from build123d import *

# Parameters (mm, degrees)
SKETCH_5_W           = 60
SKETCH_5_H           = 115
EXTRUDE_2_DEPTH      = 20
SKETCH_1_R           = 1.05
CUT_EXTRUDE_4_DEPTH  = 20
SKETCH_6_R           = 5
EXTRUDE_3_DEPTH      = 13
SKETCH_22_W          = 21
SKETCH_22_H          = 21
CUT_EXTRUDE_9_DEPTH  = 17
SKETCH_22_6_W        = 21
SKETCH_22_6_H        = 21
CUT_EXTRUDE_10_DEPTH = 17


with BuildPart() as part:
    # Sketch 5 → Extrude 2 (new body)
    with BuildSketch(Plane.XY):
        with Locations((85.095319229, -3)):
            Rectangle(SKETCH_5_W, SKETCH_5_H)
    extrude(amount=EXTRUDE_2_DEPTH)

    # Sketch 1 → Cut-Extrude 4 (cut)
    with BuildSketch(Plane.XY):
        with Locations((59.19, 1.7)):
            Circle(SKETCH_1_R)
        with Locations((106.81, 1.7)):
            Circle(SKETCH_1_R)
        with Locations((106.81, -7.7)):
            Circle(SKETCH_1_R)
        with Locations((59.19, -7.7)):
            Circle(SKETCH_1_R)
        Polygon((55, -3), (55, 0), (62, 0), (62, 7.5), (104, 7.5), (104, -13.5), (62, -13.5), (62, -6), (55, -6), align=None)
    extrude(amount=CUT_EXTRUDE_4_DEPTH, mode=Mode.SUBTRACT)

    # Sketch 6 → Extrude 3 (add)
    with BuildSketch(Plane(origin=(115, 0, 0), x_dir=(0, 0, -1), z_dir=(1, 0, 0))):
        with Locations((-10, 44.5)):
            Circle(SKETCH_6_R)
        with Locations((-10, 29.5)):
            Circle(SKETCH_6_R)
        with Locations((-10, -35.5)):
            Circle(SKETCH_6_R)
        with Locations((-10, -50.5)):
            Circle(SKETCH_6_R)
    extrude(amount=EXTRUDE_3_DEPTH)

    # Sketch 22 → Cut-Extrude 9 (cut)
    with BuildSketch(Plane.XY):
        with Locations((85, 37.5)):
            Rectangle(SKETCH_22_W, SKETCH_22_H)
    extrude(amount=CUT_EXTRUDE_9_DEPTH, mode=Mode.SUBTRACT)

    # Sketch 22_6 → Cut-Extrude 10 (cut)
    with BuildSketch(Plane.XY):
        with Locations((85, -43.5)):
            Rectangle(SKETCH_22_6_W, SKETCH_22_6_H)
    extrude(amount=CUT_EXTRUDE_10_DEPTH, mode=Mode.SUBTRACT)


solid = part.part
Verification items for the finished model (mm, model axes). A direction names the side the tool comes from. Coordinates: 2 decimals unless noted, no trailing zeros. Order: outer loops, then holes, each group sorted by start corner. A loop starts at its lowest first (then second) coordinate and runs counter-clockwise, first axis right, second up. Notation, with made-up numbers: M -24,2 L -4,2 A22 cw -4,24 Z; hole C 11.25,54 d7. An arc over 180 degrees is marked long. Write each question's results on one line, items separated by ' | '.
1) Section check B-B on z = 3.75. Record the cut outline in (x, y), plus the area to 3 significant figures.
Solved:
outline: M 55.1,-60.5 L 115.1,-60.5 L 115.1,54.5 L 55.1,54.5 L 55.1,0 L 62,0 L 62,7.5 L 104,7.5 L 104,-13.5 L 62,-13.5 L 62,-6 L 55.1,-6 Z; hole C 59.19,-7.7 d2.1; hole C 59.19,1.7 d2.1; hole M 74.5,-54 L 95.5,-54 L 95.5,-33 L 74.5,-33 Z; hole M 74.5,27 L 95.5,27 L 95.5,48 L 74.5,48 Z; hole C 106.81,-7.7 d2.1; hole C 106.81,1.7 d2.1 | area: 5,080 mm²
2) Gauge pin test, flat ends, axial feed: pin 1 Ø2 at (y, z) = (-9, 12) entering from +X; pin 2 Ø5 at (x, y) = (93.5, -45) entering from -Z; pin 3 Ø10 at (x, y) = (74.5, -4.5) entering from -Z. Record the tip position at first contact, or that the pin passes through.
Solved:
pin 1: stops at x = 115.1 | pin 2: stops at z = 0 | pin 3: passes through
3) Release check for a two-part mould opening along Y. For faces 1 (the face through (58.14, -7.65, 9.86)), 2 (the face through (74.5, 37, 8)), 3 (the face through (85, 54.5, 10)), 4 (the face through (128, -50, 10)) record: pulls with the +Y half, pulls with the -Y half, needs draft (parallel to the pull), parting line crosses it, or undercut.
Solved:
face 1: undercut | face 2: undercut | face 3: pulls with the +Y half | face 4: needs draft
4) Section check D-D on z = 13. Give the number of separate pieces and of enclosed holes in the cut face, plus the area to 3 significant figures.
Solved:
separate pieces: 1 | enclosed holes: 6 | area: 5,490 mm²
5) Access from +Z, -Z, +X, -X, +Y, -Y to the whole of each face (thin tool, end or side, straight path). Record for faces 5 (the face through (83, -13.5, 10)), 6 (the face through (58, 0, 10)), 7 (the face through (95.5, -44, 8)), 8 (the face through (121.457, 48.716, 7.312)).
Solved:
face 5: +Z, -Z | face 6: +Z, -Z, -X | face 7: -Z | face 8: +X
6) Section check A-A on x = 90.5. Record the cut outline in (y, z), plus the area to 3 significant figures.
Solved:
outline: M -60.5,0 L -54,0 L -54,17 L -33,17 L -33,0 L -13.5,0 L -13.5,20 L -60.5,20 Z; M 7.5,0 L 27,0 L 27,17 L 48,17 L 48,0 L 54.5,0 L 54.5,20 L 7.5,20 Z | area: 1,170 mm²
7) Scan lines: line 1 along Y through (x, z) = (59.19, 15.75); line 2 along Y through (x, z) = (84.5, 11.5); line 3 along Y through (x, z) = (106.81, 4.25). Record each from-to range of solid material in increasing order. Write a range as [from, to].
Solved:
line 1: y = [-60.5, -8.75], [-6.65, -6], [0, 0.65], [2.75, 54.5] | line 2: y = [-60.5, -54], [-33, -13.5], [7.5, 27], [48, 54.5] | line 3: y = [-60.5, -8.75], [-6.65, 0.65], [2.75, 54.5]
8) Section check C-C on y = 29.5. Record the cut outline in (x, z), plus the area to 3 significant figures.
Solved:
outline: M 55.1,0 L 74.5,0 L 74.5,17 L 95.5,17 L 95.5,0 L 115.1,0 L 115.1,5 L 128,5 L 128,15 L 115.1,15 L 115.1,20 L 55.1,20 Z | area: 972 mm²
